```python
from build123d import *

# Parameters (mm, degrees)
F1_DEPTH  = 6.35
F2_DEPTH  = 101.6
F3_DEPTH  = 25.4
F4_DEPTH  = 25.4
F6_DEPTH  = 76.2
F7_W      = 82.55
F7_H      = 19.05
F8_DEPTH  = 25.4
F9_W      = 82.55
F9_H      = 19.05
F10_DEPTH = 25.4


with BuildPart() as f1:
    # F0 (on Top) → F1 (new body)
    with BuildSketch(Plane.XY):
        Polygon((177.8, 0), (0, 0), (0, -177.8), (6.35, -177.8), (6.35, -6.35), (177.8, -6.35), align=None)
        Polygon((6.35, -6.35), (6.35, -177.8), (38.1, -177.8), (38.1, -37.5833287835), (177.8, -37.5833287835), (177.8, -6.35), align=None)
        Polygon((38.1, -37.5833287835), (38.1, -177.8), (44.45, -177.8), (44.45, -44.45), (177.8, -44.45), (177.8, -37.5833287835), align=None)
    extrude(amount=F1_DEPTH)

    # F0 (on Top) → F2 (join)
    with BuildSketch(Plane.XY):
        Polygon((177.8, 0), (0, 0), (0, -177.8), (6.35, -177.8), (6.35, -6.35), (177.8, -6.35), align=None)
        Polygon((38.1, -37.5833287835), (38.1, -177.8), (44.45, -177.8), (44.45, -44.45), (177.8, -44.45), (177.8, -37.5833287835), align=None)
    extrude(amount=-F2_DEPTH)

    # F3 (add): a face of the model
    f3_faces = [f1.faces().sort_by_distance(p)[0] for p in [
        (111.125, -44.45, -47.625),
    ]]
    extrude(f3_faces, amount=F3_DEPTH)

    # F4 (add): a face of the model
    f4_faces = [f1.faces().sort_by_distance(p)[0] for p in [
        (44.45, -123.825, -47.625),
    ]]
    extrude(f4_faces, amount=F4_DEPTH)

    # F5 (on face) → F6 (cut)
    with BuildSketch(Plane(origin=(0, 0, -101.6), x_dir=(1, 0, 0), z_dir=(0, 0, -1))):
        Polygon((69.85, 177.8), (44.45, 177.8), (44.45, 43.9333287835), (177.8, 43.9333287835), (177.8, 69.85), (69.85, 69.85), align=None)
    extrude(amount=-F6_DEPTH, mode=Mode.SUBTRACT)

    # F7 (on face) → F8 (cut)
    with BuildSketch(Plane.YZ.offset(69.85)):
        with Locations((-123.825, -9.525)):
            Rectangle(F7_W, F7_H)
    extrude(amount=-F8_DEPTH, mode=Mode.SUBTRACT)

    # F9 (on face) → F10 (cut)
    with BuildSketch(Plane.XZ.offset(69.85)):
        with Locations((123.825, -9.525)):
            Rectangle(F9_W, F9_H)
    extrude(amount=-F10_DEPTH, mode=Mode.SUBTRACT)


solid = f1.part
```
CAD build for the part. Positions are in the model's coordinates, mm. A direction names the side the tool comes from. Coordinates: 2 decimals unless noted, no trailing zeros. Order: outer loops, then holes, each group sorted by start corner. A loop starts at its lowest first (then second) coordinate and runs counter-clockwise, first axis right, second up.
(1) Saw through at B-B, the plane x = 63. Write the cut outline in (y, z), and give its area (3 significant figures).
Solution:
outline: (-177.8, -25.4) - (-43.93, -25.4) - (-43.93, -101.6) - (-37.58, -101.6) - (-37.58, 0) - (-6.35, 0) - (-6.35, -101.6) - (0, -101.6) - (0, 6.35) - (-177.8, 6.35) - close; hole (-165.1, -19.05) - (-82.55, -19.05) - (-82.55, 0) - (-165.1, 0) - close
area: 4,250 mm2
(2) Which spindle directions (+Z, -Z, +X, -X, +Y, -Y) get a long thin tool onto all of the face, cutting with end or side? Do faces 5 (the face through (57, -124, -19.05)), 6 (the face through (66, -82, -25.4)), 7 (the face through (123, -57, 0)), 8 (the face through (6.35, -93, -50)), 9 (the face through (91, -6.35, -50)). Say none if no direction does.
Solution:
face 5: +X
face 6: -Z, +X, -Y
face 7: -Y
face 8: -Z, -Y
face 9: -Z, +X
(3) Pin check, flat tips, straight feed: pin 1 Ø8 at (x, z) = (138, -80) entering from -Y; pin 2 Ø9.5 at (y, z) = (-107.5, -10.5) entering from +X; pin 3 Ø23 at (y, z) = (-101.5, -65.5) entering from +X. Stop position of each tip, or through.
Solution:
pin 1: stops at y = -43.93
pin 2: stops at x = 44.45
pin 3: stops at x = 44.45
(4) Saw through at C-C, the plane y = -64.5. Write the cut outline in (x, z).
Solution:
outline: (0, -101.6) - (6.35, -101.6) - (6.35, 0) - (38.1, 0) - (38.1, -101.6) - (44.45, -101.6) - (44.45, -25.4) - (177.8, -25.4) - (177.8, 6.35) - (0, 6.35) - close; hole (82.55, -19.05) - (165.1, -19.05) - (165.1, 0) - (82.55, 0) - close
(5) Saw through at A-A, the plane z = -6.5. Write the cut outline in (x, y), and give its area (3 significant figures).
Solution:
outline: (0, -177.8) - (6.35, -177.8) - (6.35, -6.35) - (177.8, -6.35) - (177.8, 0) - (0, 0) - close; (38.1, -177.8) - (69.85, -177.8) - (69.85, -165.1) - (44.45, -165.1) - (44.45, -82.55) - (69.85, -82.55) - (69.85, -69.85) - (82.55, -69.85) - (82.55, -44.45) - (165.1, -44.45) - (165.1, -69.85) - (177.8, -69.85) - (177.8, -37.58) - (38.1, -37.58) - close
area: 5,960 mm2
(6) Mould opens along X. For faces 1 (the face through (57, -124, 0)), 2 (the face through (69.85, -125, 1)), 3 (the face through (165.1, -57, -10)), 4 (the face through (82.55, -57, -10)) say: released by +X, released by -X, zero draft, split by the parting line, or undercut.
Solution:
face 1: zero draft
face 2: released by +X
face 3: undercut
face 4: undercut
(7) Drill centre lines: L1, parallel to Z at x = 146.5, y = -46; L2, parallel to Y at x = 129.5, z = -43.5; L3, parallel to X at y = -115, z = -50. Where is each one in solid material? Low to high.
Solution:
L1: z = -25.4 to -19.05, 0 to 6.35
L2: y = -43.93 to -37.58, -6.35 to 0
L3: x = 0 to 6.35, 38.1 to 44.45
(8) Saw through at D-D, the plane y = -136. Write the cut outline in (x, z), and give its area (3 significant figures).
Solution:
outline: (0, -101.6) - (6.35, -101.6) - (6.35, 0) - (38.1, 0) - (38.1, -101.6) - (44.45, -101.6) - (44.45, -25.4) - (69.85, -25.4) - (69.85, -19.05) - (44.45, -19.05) - (44.45, 0) - (69.85, 0) - (69.85, 6.35) - (0, 6.35) - close
area: 1,900 mm2
